The model under review builds one solid part; all positions refer to its coordinate system, in mm. Face numbers are marked on the shaded views. A direction names the side the tool comes from. Round coordinates to 2 decimals unless told otherwise and drop trailing zeros. Order: outer loops, then holes, each group sorted by start corner. A loop starts at its lowest first (then second) coordinate and runs counter-clockwise, first axis right, second up. Notation, with made-up numbers: (68, -7.75) -> (79, -7.75) arc R22 cw to (79, -0.75) -> close; hole circle Ø5 at (12.25, 60.25). An arc over 180 degrees is marked (long way). Use a Markdown table: item, result. Add a question column.
```python
from build123d import *

# Parameters (mm, degrees)
SKETCH1_W           = 70
SKETCH1_H           = 46
SKETCH1_R           = 11
BOSS_EXTRUDE1_DEPTH = 8
SKETCH2_W           = 70
SKETCH2_H           = 46
SKETCH2_R           = 21.5
BOSS_EXTRUDE2_DEPTH = 6
SKETCH3_R           = 2.25
CUT_EXTRUDE1_DEPTH  = 9
CUT_EXTRUDE2_DEPTH  = 3.2
FILLET1_R           = 5
SKETCH6_R           = 2.25
CUT_EXTRUDE3_DEPTH  = 15


with BuildPart() as part:
    # Sketch1 → Boss-Extrude1 (new body)
    with BuildSketch(Plane(origin=(0, 0, 0), x_dir=(1, 0, 0), z_dir=(0, 1, 0))):
        Rectangle(SKETCH1_W, SKETCH1_H)
        Circle(SKETCH1_R, mode=Mode.SUBTRACT)
    extrude(amount=BOSS_EXTRUDE1_DEPTH)

    # Sketch2 → Boss-Extrude2 (add)
    with BuildSketch(Plane(origin=(0, 8, 0), x_dir=(1, 0, 0), z_dir=(0, 1, 0))):
        Rectangle(SKETCH2_W, SKETCH2_H)
        Circle(SKETCH2_R, mode=Mode.SUBTRACT)
    extrude(amount=BOSS_EXTRUDE2_DEPTH)

    # Sketch3 → Cut-Extrude1 (cut, through all)
    with BuildSketch(Plane(origin=(0, 8, 0), x_dir=(1, 0, 0), z_dir=(0, 1, 0))):
        with Locations((-11.730749234, 10.880694942)):
            Circle(SKETCH3_R)
        with Locations((11.730749234, 10.880694942)):
            Circle(SKETCH3_R)
        with Locations((11.730749234, -10.880694942)):
            Circle(SKETCH3_R)
        with Locations((-11.730749234, -10.880694942)):
            Circle(SKETCH3_R)
    extrude(amount=-CUT_EXTRUDE1_DEPTH, mode=Mode.SUBTRACT)

    # Sketch5 → Cut-Extrude2 (cut)
    with BuildSketch(Plane.XZ):
        Polygon((-12.629361921, 14.820977745), (-15.592440583, 12.072614928), (-14.693827896, 8.132332124), (-10.832136547, 6.940412138), (-7.869057884, 9.688774955), (-8.767670572, 13.629057759), align=None)
        Polygon((-10.832136547, -6.940412138), (-14.693827896, -8.132332124), (-15.592440583, -12.072614928), (-12.629361921, -14.820977745), (-8.767670572, -13.629057759), (-7.869057884, -9.688774955), align=None)
        Polygon((10.832136547, -6.940412138), (7.869057884, -9.688774955), (8.767670572, -13.629057759), (12.629361921, -14.820977745), (15.592440583, -12.072614928), (14.693827896, -8.132332124), align=None)
        Polygon((7.869057884, 9.688774955), (10.832136547, 6.940412138), (14.693827896, 8.132332124), (15.592440583, 12.072614928), (12.629361921, 14.820977745), (8.767670572, 13.629057759), align=None)
    extrude(amount=-CUT_EXTRUDE2_DEPTH, mode=Mode.SUBTRACT)

    # Fillet1
    fillet1_edges = [part.edges().sort_by_distance(p)[0] for p in [
        (35, 7, 23),
        (-35, 7, 23),
        (-35, 7, -23),
        (35, 7, -23),
    ]]
    fillet(fillet1_edges, radius=FILLET1_R)

    # Sketch6 → Cut-Extrude3 (cut, through all)
    with BuildSketch(Plane(origin=(0, 14, 0), x_dir=(1, 0, 0), z_dir=(0, 1, 0))):
        with Locations((-30, 18)):
            Circle(SKETCH6_R)
        with Locations((-30, -18)):
            Circle(SKETCH6_R)
        with Locations((30, -18)):
            Circle(SKETCH6_R)
        with Locations((30, 18)):
            Circle(SKETCH6_R)
        with Locations((-30, 6)):
            Circle(SKETCH6_R)
        with Locations((-30, -6)):
            Circle(SKETCH6_R)
        with Locations((30, -6)):
            Circle(SKETCH6_R)
        with Locations((30, 6)):
            Circle(SKETCH6_R)
    extrude(amount=-CUT_EXTRUDE3_DEPTH, mode=Mode.SUBTRACT)


solid = part.part
```
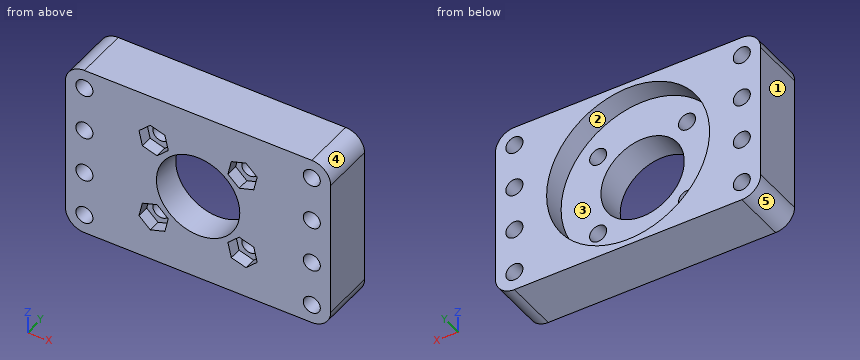
Q1. Machinability: for the marked faces 1 and 2, which of the approach directions +Z, -Z, +X, -X, +Y, -Y give a long, thin tool a straight path to every point of the face, cutting with its end or side? Answer none if there is none.
Q2. Mouldability with a two-part tool opening along X and no side actions: class the marked faces 3, 4 and 5 as pulls with the +X half, pulls with the -X half, needs draft (parallel to the pull), parting line crosses it, or undercut.
Q3. Add section C-C (y = 1). State how many separate pieces and enclosed holes the cut face has, then the cut area to 3 significant figures.
Q4. Add section A-A (x = 0). Write out the cut boundary in (y, z), then the cut area to 3 significant figures.
Q5. Insertion check: pin 1 (4 mm diameter, centred on x = 12.5, z = 12, fed in from -Y). The pin has a flat end and moves straight along its axis. Give the tip position at first contact, or say it passes through.
Q6. Add section B-B (z = 2). Write out the cut boundary in (x, y), then the cut area to 3 significant figures.
Q7. Wall thickness on line 1 (X direction, y = 4, z = 18); line 2 (Z direction, x = -30, y = 7.25); line 3 (Z direction, x = 0, y = 9): over which ranges is each line inside the solid? List them lowest first. Write a range as [from, to].
Report:
| question | item | result |
|---|---|---|
| 1 | face 1 | +Z, -Z, -X, +Y, -Y |
| 1 | face 2 | +Y |
| 2 | face 3 | undercut |
| 2 | face 4 | pulls with the +X half |
| 2 | face 5 | pulls with the -X half |
| 3 | separate pieces | 1 |
| 3 | enclosed holes | 13 |
| 3 | area | 2,520 mm² |
| 4 | outline | (0, -23) -> (14, -23) -> (14, -21.5) -> (8, -21.5) -> (8, -11) -> (0, -11) -> close; (0, 11) -> (8, 11) -> (8, 21.5) -> (14, 21.5) -> (14, 23) -> (0, 23) -> close |
| 4 | area | 210 mm² |
| 5 | pin 1 | stops at y = 3.2 |
| 6 | outline | (-35, 0) -> (-10.82, 0) -> (-10.82, 8) -> (-21.41, 8) -> (-21.41, 14) -> (-35, 14) -> close; (10.82, 0) -> (35, 0) -> (35, 14) -> (21.41, 14) -> (21.41, 8) -> (10.82, 8) -> close |
| 6 | area | 550 mm² |
| 7 | line 1 | x = [-35, -32.25], [-27.75, 27.75], [32.25, 35] |
| 7 | line 2 | z = [-23, -20.25], [-15.75, -8.25], [-3.75, 3.75], [8.25, 15.75], [20.25, 23] |
| 7 | line 3 | z = [-23, -21.5], [21.5, 23] |
